Verification items for this drawing (mm, ordinates from the low corner). Give positions to 0.01 mm unless a question says otherwise; leave off trailing zeros. Order: outer loops, then holes, each group sorted by start corner. A loop starts at its lowest first (then second) coordinate and runs counter-clockwise, first axis right, second up. Notation, with made-up numbers: M 78,0.25 L 83,0.25 A8 cw 83,8.25 Z; hole C -19,30 d3. An arc over 180 degrees is marked long. One line per question, with ' | ' between items. Start each with the question number.
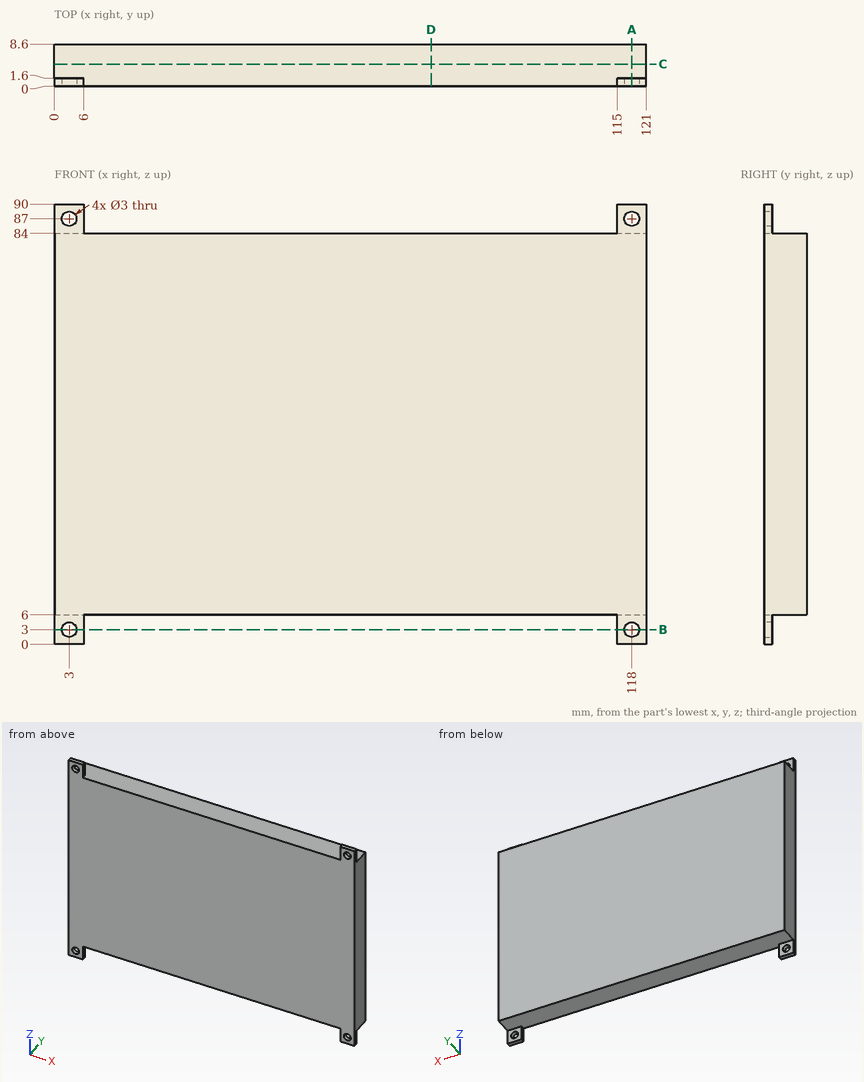
Item 1: Depth check by flat-ended pin: pin 1 (2.5 mm diameter, centred on x = 43.5, y = 5.5, fed in from -Z); pin 2 (4 mm diameter, centred on x = 76, y = 6, fed in from +Z); pin 3 (1.8 mm diameter, centred on x = 116.5, z = 2, fed in from +Y). Enter the tip coordinate at first touch or a pass-through.
Item 2: Material ranges on line 1 along X through (y, z) = (1.1, 3); line 2 along Z through (x, y) = (29.5, 5.5), recorded low to high.
Item 3: Cross-section at A-A, the plane x = 118. Record the cut outline in (y, z).
Item 4: Cross-section at D-D, the plane x = 77. Record the cut outline in (y, z), plus the area to 3 significant figures.
Item 5: Cross-section at C-C, the plane y = 4.5. Record the cut outline in (x, z).
Item 6: Cross-section at B-B, the plane z = 3. Record the cut outline in (x, y), plus the area to 3 significant figures.
Outcome:
1) pin 1: stops at z = 6 | pin 2: stops at z = 84 | pin 3: stops at y = 1.6
2) line 1: x = 0 to 1.5, 4.5 to 6, 115 to 116.5, 119.5 to 121 | line 2: z = 6 to 84
3) outline: M 0,0 L 1.6,0 L 1.6,1.5 L 0,1.5 Z; M 0,4.5 L 1.6,4.5 L 1.6,6 L 8.6,6 L 8.6,84 L 1.6,84 L 1.6,85.5 L 0,85.5 Z; M 0,88.5 L 1.6,88.5 L 1.6,90 L 0,90 Z
4) outline: M 0,6 L 8.6,6 L 8.6,84 L 0,84 Z | area: 671 mm²
5) outline: M 0,6 L 121,6 L 121,84 L 0,84 Z
6) outline: M 0,0 L 1.5,0 L 1.5,1.6 L 0,1.6 Z; M 4.5,0 L 6,0 L 6,1.6 L 4.5,1.6 Z; M 115,0 L 116.5,0 L 116.5,1.6 L 115,1.6 Z; M 119.5,0 L 121,0 L 121,1.6 L 119.5,1.6 Z | area: 9.60 mm²
